```python
from build123d import *

# Parameters (mm, degrees)
F0_W     = 128.6
F0_H     = 12.2
F0_W_2   = 13.5
F0_H_2   = 6
F1_DEPTH = 5
F0_H_3   = 1.6
F2_DEPTH = 2.5


with BuildPart() as f1:
    # F0 (on Front) → F1 (new body)
    with BuildSketch(Plane.XZ):
        with Locations((0, -0.8)):
            Rectangle(F0_W, F0_H)
        with Locations((-30, 0)):
            Rectangle(F0_W_2, F0_H_2, mode=Mode.SUBTRACT)
        with Locations((-10, 0)):
            Rectangle(F0_W_2, F0_H_2, mode=Mode.SUBTRACT)
        with Locations((10, 0)):
            Rectangle(F0_W_2, F0_H_2, mode=Mode.SUBTRACT)
        with Locations((30, 0)):
            Rectangle(F0_W_2, F0_H_2, mode=Mode.SUBTRACT)
    extrude(amount=F1_DEPTH)

    # F0 (on Front) → F2 (join)
    with BuildSketch(Plane.XZ):
        with BuildLine():
            Line((-64.3, -6.9), (-64.3, 5.3))
            ThreePointArc((-64.3, 5.3), (-65.3, 4.3), (-66.3, 5.3))
            Line((-66.3, 5.3), (-70.25, 5.3))
            Line((-70.25, 5.3), (-70.25, -6.9))
            Line((-70.25, -6.9), (-64.3, -6.9))
        make_face()
        with Locations((0, 6.1)):
            Rectangle(F0_W, F0_H_3)
        with BuildLine():
            ThreePointArc((66.3, 5.3), (65.3, 4.3), (64.3, 5.3))
            Line((64.3, 5.3), (64.3, -6.9))
            Line((64.3, -6.9), (70.25, -6.9))
            Line((70.25, -6.9), (70.25, 5.3))
            Line((70.25, 5.3), (66.3, 5.3))
        make_face()
    extrude(amount=F2_DEPTH)


solid = f1.part
```
The model under review builds one solid part; all positions refer to its coordinate system, in mm. A direction names the side the tool comes from. Round coordinates to 2 decimals unless told otherwise and drop trailing zeros. Order: outer loops, then holes, each group sorted by start corner. A loop starts at its lowest first (then second) coordinate and runs counter-clockwise, first axis right, second up. Notation, with made-up numbers: (-23, -10.75) - (-13, -10.75) arc R33 ccw to (-13, 18.25) - close; hole circle Ø8 at (41, 16). An arc over 180 degrees is marked (long way). Answer in a Markdown table with one row per item.
(1) Clearance check with flat-ended pins moving along their axes: P1, Ø1.5, axis at y = -4, z = 5.5, coming from the +X side; P2, Ø1.3, axis at x = -11, z = 6, coming from the -Y side; P3, Ø2, axis at x = -49, z = -0.5, coming from the +Y side; P4, Ø0.5, axis at y = -1, z = 6, coming from the -X side. State where each tip first meets the part, or that it passes through.
Result set:
| item | result |
|---|---|
| P1 | stops at x = 64.3 |
| P2 | stops at y = -2.5 |
| P3 | stops at y = 0 |
| P4 | stops at x = -64.3 |
(2) Take a section at B-B on y = -3.6. Write out the cut boundary in (x, z), plus the area to 3 significant figures.
Result set:
| item | result |
|---|---|
| outline | (-64.3, -6.9) - (64.3, -6.9) - (64.3, 5.3) - (-64.3, 5.3) - close; hole (-36.75, -3) - (-23.25, -3) - (-23.25, 3) - (-36.75, 3) - close; hole (-16.75, -3) - (-3.25, -3) - (-3.25, 3) - (-16.75, 3) - close; hole (3.25, -3) - (16.75, -3) - (16.75, 3) - (3.25, 3) - close; hole (23.25, -3) - (36.75, -3) - (36.75, 3) - (23.25, 3) - close |
| area | 1,240 mm2 |
(3) Take a section at C-C on x = -10.5. Write out the cut boundary in (y, z).
Result set:
| item | result |
|---|---|
| outline | (-5, -6.9) - (0, -6.9) - (0, -3) - (-5, -3) - close; (-5, 3) - (0, 3) - (0, 6.9) - (-2.5, 6.9) - (-2.5, 5.3) - (-5, 5.3) - close |
(4) Take a section at A-A on z = 0.5. Write out the cut boundary in (x, y), plus the area to 3 significant figures.
Result set:
| item | result |
|---|---|
| outline | (-70.25, -2.5) - (-64.3, -2.5) - (-64.3, -5) - (-36.75, -5) - (-36.75, 0) - (-70.25, 0) - close; (-23.25, -5) - (-16.75, -5) - (-16.75, 0) - (-23.25, 0) - close; (-3.25, -5) - (3.25, -5) - (3.25, 0) - (-3.25, 0) - close; (16.75, -5) - (23.25, -5) - (23.25, 0) - (16.75, 0) - close; (36.75, -5) - (64.3, -5) - (64.3, -2.5) - (70.25, -2.5) - (70.25, 0) - (36.75, 0) - close |
| area | 403 mm2 |
(5) For line 1 (X direction, y = -3.95, z = -1.25); line 2 (X direction, y = -1.6, z = -1.25); line 3 (Z direction, x = 36.5, y = -3.8), list the stretches that pass through material, from the lowest coordinate up. Write a range as from..to.
Result set:
| item | result |
|---|---|
| line 1 | x = -64.3..-36.75, -23.25..-16.75, -3.25..3.25, 16.75..23.25, 36.75..64.3 |
| line 2 | x = -70.25..-36.75, -23.25..-16.75, -3.25..3.25, 16.75..23.25, 36.75..70.25 |
| line 3 | z = -6.9..-3, 3..5.3 |
(6) Take a section at D-D on x = 21. Write out the cut boundary in (y, z).
Result set:
| item | result |
|---|---|
| outline | (-5, -6.9) - (0, -6.9) - (0, 6.9) - (-2.5, 6.9) - (-2.5, 5.3) - (-5, 5.3) - close |
(7) Mouldability with a two-part tool opening along X and no side actions: class faces 1 (the face through (-30, -2, 3)), 2 (the face through (-1, 0, 0)), 3 (the face through (70.25, -1, -1)), 4 (the face through (-23.25, -2, 0)) as released by +X, released by -X, zero draft, split by the parting line, or undercut.
Result set:
| item | result |
|---|---|
| face 1 | undercut |
| face 2 | zero draft |
| face 3 | released by +X |
| face 4 | undercut |
(8) Machinability: for faces 5 (the face through (-3.25, -2, 0)), 6 (the face through (-68, -1, 5.3)), 7 (the face through (-64.3, -4, -1)), which of the approach directions +Z, -Z, +X, -X, +Y, -Y give a long, thin tool a straight path to every point of the face, cutting with its end or side? Answer none if there is none.
Result set:
| item | result |
|---|---|
| face 5 | +Y, -Y |
| face 6 | +Z, -X, +Y, -Y |
| face 7 | +Z, -Z, -X, -Y |
